```python
from build123d import *

# Parameters (mm, degrees)
SALIENTE_EXTRUIR1_DEPTH = 3
REDONDEO1_R             = 5
REDONDEO2_R             = 10
CROQUIS2_R              = 1.5
CROQUIS2_R_2            = 5
CROQUIS2_R_3            = 1
CROQUIS2_W              = 35
CROQUIS2_H              = 12
CROQUIS2_W_2            = 70
CROQUIS2_H_2            = 2
CROQUIS2_W_3            = 3
CROQUIS2_H_3            = 20
CORTAR_EXTRUIR1_DEPTH   = 10
CHAFL_N1_SIZE           = 10
REDONDEO3_R             = 5


with BuildPart() as part:
    # Croquis1 → Saliente-Extruir1 (new body)
    with BuildSketch(Plane.XY):
        Polygon((70, 0), (-70, 0), (-70, 70), (-30, 70), (-15, 140), (-25, 140), (-25, 160), (-50, 160), (-50, 190), (50, 190), (50, 160), (25, 160), (25, 140), (15, 140), (30, 70), (70, 70), align=None)
    extrude(amount=SALIENTE_EXTRUIR1_DEPTH)

    # Redondeo1
    redondeo1_edges = [part.edges().sort_by_distance(p)[0] for p in [
        (-15, 140, 1.5),
        (-50, 160, 1.5),
        (50, 160, 1.5),
        (15, 140, 1.5),
    ]]
    fillet(redondeo1_edges, radius=REDONDEO1_R)

    # Redondeo2
    redondeo2_edges = [part.edges().sort_by_distance(p)[0] for p in [
        (-70, 70, 1.5),
        (-30, 70, 1.5),
        (30, 70, 1.5),
        (70, 70, 1.5),
    ]]
    fillet(redondeo2_edges, radius=REDONDEO2_R)

    # Croquis2 → Cortar-Extruir1 (cut)
    with BuildSketch(Plane.XY.offset(3)):
        with Locations((-55, 10)):
            Circle(CROQUIS2_R)
        with Locations((-55, 30)):
            Circle(CROQUIS2_R)
        with Locations((55, 10)):
            Circle(CROQUIS2_R)
        with Locations((55, 30)):
            Circle(CROQUIS2_R)
        with Locations((34.95, 165)):
            Circle(CROQUIS2_R)
        with Locations((-0.20543979, 151.386853188)):
            Circle(CROQUIS2_R_2)
        with Locations((-7.65543979, 151.386853188)):
            Circle(CROQUIS2_R_3)
        with Locations((7.34456021, 151.386853188)):
            Circle(CROQUIS2_R_3)
        with Locations((-65, 5)):
            Circle(CROQUIS2_R)
        with Locations((-60, 60)):
            Circle(CROQUIS2_R)
        with Locations((65, 5)):
            Circle(CROQUIS2_R)
        with Locations((60, 60)):
            Circle(CROQUIS2_R)
        with Locations((0, 5)):
            Circle(CROQUIS2_R)
        with Locations((0, 60)):
            Circle(CROQUIS2_R)
        with Locations((-19, 65)):
            Circle(CROQUIS2_R)
        with Locations((17.5, 65)):
            Circle(CROQUIS2_R)
        with Locations((-19, 101.5)):
            Circle(CROQUIS2_R)
        with Locations((17.5, 101.5)):
            Circle(CROQUIS2_R)
        with Locations((-34.95, 165)):
            Circle(CROQUIS2_R)
        with Locations((0.45, 166.017006834)):
            Rectangle(CROQUIS2_W, CROQUIS2_H)
        with Locations((0, 183)):
            Rectangle(CROQUIS2_W_2, CROQUIS2_H_2)
        with Locations((-44, 20)):
            Rectangle(CROQUIS2_W_3, CROQUIS2_H_3)
        with Locations((44, 20)):
            Rectangle(CROQUIS2_W_3, CROQUIS2_H_3)
    extrude(amount=-CORTAR_EXTRUIR1_DEPTH, mode=Mode.SUBTRACT)

    # Chaflán1
    chafl_n1_edges = [part.edges().sort_by_distance(p)[0] for p in [
        (-50, 190, 1.5),
        (50, 190, 1.5),
    ]]
    chamfer(chafl_n1_edges, length=CHAFL_N1_SIZE)

    # Redondeo3
    redondeo3_edges = [part.edges().sort_by_distance(p)[0] for p in [
        (40, 190, 1.5),
        (-40, 190, 1.5),
    ]]
    fillet(redondeo3_edges, radius=REDONDEO3_R)


solid = part.part
```
Here's how the part is built. I have some questions about the finished solid (model axes, mm). A direction names the side the tool comes from. Coordinates: 2 decimals unless noted, no trailing zeros. Order: outer loops, then holes, each group sorted by start corner. A loop starts at its lowest first (then second) coordinate and runs counter-clockwise, first axis right, second up. Notation, with made-up numbers: (-17, 51) -> (30, 51) arc R10 ccw to (30, 55) -> close; hole circle Ø5 at (38.5, 13). An arc over 180 degrees is marked (long way). Return JSON: item names as keys, results as strings.
1) If I drill on probe 1 along Y at (x, z) = (-14.5, 2.15); probe 2 along X at (y, z) = (28, 0.3); probe 3 along Y at (x, z) = (0, 2.2), over which ranges is the centre line in solid material (lowest first)?
Conclusion:
{"probe 1": "y = 0 to 160.02, 172.02 to 182, 184 to 190", "probe 2": "x = -70 to -45.5, -42.5 to 42.5, 45.5 to 70", "probe 3": "y = 0 to 3.5, 6.5 to 58.5, 61.5 to 146.39, 156.38 to 160.02, 172.02 to 182, 184 to 190"}
2) If we section it at B-B on y = 116: List the corners of the cut face in (x, z) for me.
Conclusion:
{"outline": "(-20.14, 0) -> (20.14, 0) -> (20.14, 3) -> (-20.14, 3) -> close"}
3) On a 3-axis mill with a long thin cutter (end or side, diameter ignored), from which of +Z, -Z, +X, -X, +Y, -Y can I reach the whole of each face in a straight line? I mean faces 4 (the cylindrical face through (31.872, 72.164, 1.521)), 5 (the cylindrical face through (-48, 161, 2)), 6 (the flat face through (-46, 184, 1)). Say none if no direction works.
Conclusion:
{"face 4": "+Z, -Z, +X", "face 5": "+Z, -Z, -X", "face 6": "+Z, -Z, -X, +Y"}
4) I'm going to push flat-ended pins straight in: P1, Ø0.9, axis at x = 43.5, z = 2, coming from the -Y side; P2, Ø1.5, axis at y = 151, z = 1, coming from the +X side; P3, Ø1.5, axis at x = -47.5, z = 2, coming from the +Y side. Where does each tip first touch, or does it pass through?
Conclusion:
{"P1": "stops at y = 0", "P2": "stops at x = 25", "P3": "stops at y = 183.25"}
5) If we section it at A-A on z = 1.25: State how many separate pieces and enclosed holes the cut face has, plus the area to 3 significant figures.
Conclusion:
{"separate pieces": "1", "enclosed holes": "23", "area": "16,000 mm²"}
6) Thinking about a two-plate mould opening in Y: for faces 1 (the cylindrical face through (-1.289, 146.506, 1.521)), 2 (the flat face through (1, 75, 0)), 3 (the cylindrical face through (67.15, 66.99, 1.52)), which applies, +Y half, -Y half, draft (parallel to the pull), parting line (faces both ways), or undercut?
Conclusion:
{"face 1": "undercut", "face 2": "draft", "face 3": "+Y half"}
